Geometry: final body of the model. Coordinates: model frame, mm. A direction names the side the tool comes from. Give positions to 0.01 mm unless a question says otherwise; leave off trailing zeros. Write each loop counter-clockwise with the first axis right and the second up, starting at its lowest first coordinate (ties: lowest second). Pieces come first, ordered by that corner, then holes. Notation, with made-up numbers: (16, 75) - (33, 75) arc R17 ccw to (33, 89) - close; hole circle Ø2 at (88.25, 63). An arc over 180 degrees is marked (long way). Return JSON: item names as keys, results as strings.
from build123d import *

# Parameters (mm, degrees)
SKETCH1_R           = 40.64
BOSS_EXTRUDE1_DEPTH = 53.34
FILLET1_R           = 6.35
SKETCH2_R           = 38.1
CUT_EXTRUDE1_DEPTH  = 50.8
SKETCH7_W           = 5.08
SKETCH7_H           = 57.15
BOSS_EXTRUDE3_DEPTH = 63.5
SKETCH8_W           = 12.7
SKETCH8_H           = 6.35
BOSS_EXTRUDE4_DEPTH = 6.096


with BuildPart() as part:
    # Sketch1 → Boss-Extrude1 (new body)
    with BuildSketch(Plane(origin=(0, 0, 0), x_dir=(1, 0, 0), z_dir=(0, 1, 0))):
        with Locations(Location((0, 0, 0), (0, 0, 270))):
            Circle(SKETCH1_R)
    extrude(amount=BOSS_EXTRUDE1_DEPTH)

    # Fillet1
    fillet1_edges = [part.edges().sort_by_distance(p)[0] for p in [
        (0, 0, -40.64),
    ]]
    fillet(fillet1_edges, radius=FILLET1_R)

    # Sketch2 → Cut-Extrude1 (cut)
    with BuildSketch(Plane(origin=(0, 53.34, 0), x_dir=(1, 0, 0), z_dir=(0, 1, 0))):
        with Locations(Location((0, 0, 0), (0, 0, 270))):
            Circle(SKETCH2_R)
    extrude(amount=-CUT_EXTRUDE1_DEPTH, mode=Mode.SUBTRACT)



with BuildPart() as body_2:
    # Sketch7 → Boss-Extrude3 (new body)
    with BuildSketch(Plane(origin=(-28.736819587, 0, 28.736819587), x_dir=(0.7071067811865477, 0, 0.7071067811865475), z_dir=(-0.7071067811865475, 0, 0.7071067811865477))):
        with Locations((-40.64, 34.925)):
            Rectangle(SKETCH7_W, SKETCH7_H)
    extrude(amount=-BOSS_EXTRUDE3_DEPTH)


with BuildPart() as part_1:
    add(part.part)

    add(body_2.part)  # Boss-Extrude4 merges body 2
    # Sketch8 → Boss-Extrude4 (add)
    with BuildSketch(Plane(origin=(-30.532870812, 0, -30.532870812), x_dir=(-0.7071067811865474, 0, 0.7071067811865477), z_dir=(-0.7071067811865477, 0, -0.7071067811865474))):
        with Locations((34.29, 60.325)):
            Rectangle(SKETCH8_W, SKETCH8_H)
        with Locations((34.29, 34.925)):
            Rectangle(SKETCH8_W, SKETCH8_H)
        with Locations((8.89, 60.325)):
            Rectangle(SKETCH8_W, SKETCH8_H)
        with Locations((34.29, 9.525)):
            Rectangle(SKETCH8_W, SKETCH8_H)
        with Locations((8.89, 34.925)):
            Rectangle(SKETCH8_W, SKETCH8_H)
        with Locations((8.89, 9.525)):
            Rectangle(SKETCH8_W, SKETCH8_H)
        with Locations((-16.51, 60.325)):
            Rectangle(SKETCH8_W, SKETCH8_H)
        with Locations((-16.51, 34.925)):
            Rectangle(SKETCH8_W, SKETCH8_H)
        with Locations((-16.51, 9.525)):
            Rectangle(SKETCH8_W, SKETCH8_H)
    extrude(amount=BOSS_EXTRUDE4_DEPTH)


solid = part_1.part
Q1. Mould query, pull axis Z, two halves, no side actions, for faces 6 (the flat face through (-34.45, 34.88, -30.86)), 7 (the flat face through (-43.43, 60.28, -21.88)), 8 (the flat face through (0, 0, 0)), 9 (the cylindrical face through (-23.183, 28.296, -30.235)). Classes: pulls with the +Z half, pulls with the -Z half, needs draft (parallel to the pull), parting line crosses it, or undercut.
Answer key:
{"face 6": "pulls with the -Z half", "face 7": "undercut", "face 8": "needs draft", "face 9": "undercut"}
Q2. Section query A-A, the plane z = 0. Return the cut outline in (x, y).
Answer key:
{"outline": "(-57.47, 6.35) - (-53.88, 6.35) - (-53.88, 63.5) - (-57.47, 63.5) - close; (-40.64, 6.35) arc R6.35 ccw to (-34.29, 0) - (34.29, 0) arc R6.35 ccw to (40.64, 6.35) - (40.64, 53.34) - (38.1, 53.34) - (38.1, 2.54) - (-38.1, 2.54) - (-38.1, 53.34) - (-40.64, 53.34) - close"}
Q3. Material intervals for probe 1 along Z at (x, y) = (0, 37); probe 2 along X at (y, z) = (36.5, 0); probe 3 along X at (y, z) = (33, -16.5), sorted ascending. Write a range as [from, to].
Answer key:
{"probe 1": "z = [-40.64, -38.1], [38.1, 40.64]", "probe 2": "x = [-57.47, -53.88], [-40.64, -38.1], [38.1, 40.64]", "probe 3": "x = [-44.57, -37.38], [-37.14, -34.34], [34.34, 37.14]"}
Q4. Pin query (flat end, axial travel): P1, Ø1, axis at y = 15, z = -33, coming from the +X side; P2, Ø14.5, axis at x = -37.5, z = -26.5, coming from the -Y side; P3, Ø1, axis at y = 17.5, z = 0, coming from the -X side. Return the tip coordinate at first contact, or that it passes through.
Answer key:
{"P1": "stops at x = 24.4", "P2": "stops at y = 1.75", "P3": "stops at x = -57.97"}
Q5. Section query C-C, the plane x = 0. Return the cut outline in (y, z).
Answer key:
{"outline": "(0, -34.29) arc R6.35 ccw to (6.35, -40.64) - (53.34, -40.64) - (53.34, -38.1) - (2.54, -38.1) - (2.54, 38.1) - (53.34, 38.1) - (53.34, 40.64) - (6.35, 40.64) arc R6.35 ccw to (0, 34.29) - close"}
Q6. Section query D-D, the plane y = 9.5. Return the cut outline in (x, z), plus the area to 3 significant figures.
Answer key:
{"outline": "(-63.58, -6.11) - (-54.6, -15.09) - (-50.29, -10.78) - (-41.31, -19.76) - (-45.62, -24.07) - (-36.64, -33.05) - (-32.33, -28.74) - (-23.35, -37.72) - (-27.66, -42.03) - (-18.68, -51.01) - (-10.78, -43.11) - (-16.94, -36.94) arc R40.64 ccw (long way) to (-36.94, -16.94) - (-55.68, 1.8) - close; hole circle Ø76.2 at (0, 0)", "area": "1,130 mm^2"}
Q7. Section query B-B, the plane y = 16.5. Return the cut outline in (x, z), plus the area to 3 significant figures.
Answer key:
{"outline": "(-59.27, -1.8) - (-14.37, -46.7) - (-10.78, -43.11) - (-16.94, -36.94) arc R40.64 ccw (long way) to (-36.94, -16.94) - (-55.68, 1.8) - close; hole circle Ø76.2 at (0, 0)", "area": "903 mm^2"}
Q8. Set-up query: faces 1 (the flat face through (-39, 12.7, -26)), 2 (the flat face through (-25.47, 9.48, -39.84)), 3 (the flat face through (-38, 6.35, -24)), 4 (the flat face through (-41.067, 34.969, -28.62)), 5 (the flat face through (-52.415, 9.481, -12.901)). Return all of +Z, -Z, +X, -X, +Y, -Y with unobstructed straight access to the full face (end or side cutting, diameter ignored); none if empty.
Answer key:
{"face 1": "-Z, -X", "face 2": "-X, +Y, -Y", "face 3": "-Z, -X, -Y", "face 4": "-Z, -X, +Y, -Y", "face 5": "-Z, +Y, -Y"}
